from build123d import *

# Parameters (mm, degrees)
F1_R      = 300
F2_DEPTH  = 550
F3_R      = 200
F4_DEPTH  = 150
F5_R      = 100
F6_DEPTH  = 400.001
F8_DEPTH  = 250
F10_DEPTH = 250
F12_DEPTH = 250.001
F13_R     = 60
F14_DEPTH = 250.001


with BuildPart() as f2:
    # F1 (on Top) → F2 (new body)
    with BuildSketch(Plane.XY):
        Circle(F1_R)
    extrude(amount=F2_DEPTH)

    # F3 (on face) → F4 (cut)
    with BuildSketch(Plane.XY.offset(550)):
        Circle(F3_R)
    extrude(amount=-F4_DEPTH, mode=Mode.SUBTRACT)

    # F5 (on face) → F6 (cut, through all)
    with BuildSketch(Plane.XY.offset(400)):
        Circle(F5_R)
    extrude(amount=-F6_DEPTH, mode=Mode.SUBTRACT)

    # F7 (on face) → F8 (join)
    with BuildSketch(Plane(origin=(0, 0, 0), x_dir=(1, 0, 0), z_dir=(0, 0, -1))):
        with BuildLine():
            Line((-240, -180), (-240, 180))
            Line((-240, 180), (-540, 180))
            ThreePointArc((-540, 180), (-610.710678, 150.710678), (-640, 80))
            Line((-640, 80), (-640, -80))
            ThreePointArc((-640, -80), (-610.710678, -150.710678), (-540, -180))
            Line((-540, -180), (-240, -180))
        make_face()
    extrude(amount=-F8_DEPTH)

    # F9 (on face) → F10 (join)
    with BuildSketch(Plane(origin=(0, 0, 0), x_dir=(1, 0, 0), z_dir=(0, 0, -1))):
        with BuildLine():
            Line((540, 180), (240, 180))
            Line((240, 180), (240, -180))
            Line((240, -180), (540, -180))
            ThreePointArc((540, -180), (610.710678, -150.710678), (640, -80))
            Line((640, -80), (640, 80))
            ThreePointArc((640, 80), (610.710678, 150.710678), (540, 180))
        make_face()
    extrude(amount=-F10_DEPTH)

    # F11 (on face) → F12 (cut, through all)
    with BuildSketch(Plane.XY.offset(250)):
        with BuildLine():
            Line((430, 0), (550, 0))
            ThreePointArc((550, 0), (490, 60), (430, 0))
        make_face()
        with BuildLine():
            ThreePointArc((430, 0), (490, -60), (550, 0))
            Line((550, 0), (430, 0))
        make_face()
    extrude(amount=-F12_DEPTH, mode=Mode.SUBTRACT)

    # F13 (on face) → F14 (cut, through all)
    with BuildSketch(Plane.XY.offset(250)):
        with Locations((-490, 0)):
            Circle(F13_R)
    extrude(amount=-F14_DEPTH, mode=Mode.SUBTRACT)


solid = f2.part
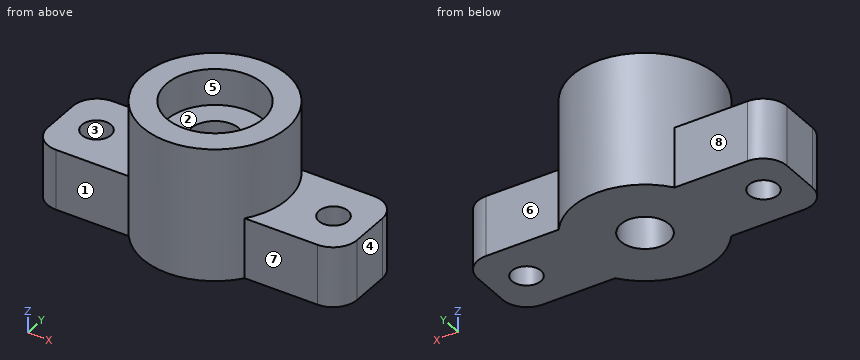
Here's how the part is built. I have some questions about the finished solid (model axes, mm). Face numbers are marked on the shaded views. A direction names the side the tool comes from. Round coordinates to 2 decimals unless told otherwise and drop trailing zeros. Order: outer loops, then holes, each group sorted by start corner. A loop starts at its lowest first (then second) coordinate and runs counter-clockwise, first axis right, second up. Notation, with made-up numbers: M 61,-6 L 79,-6 A19 ccw 79,13 Z; hole C -22.75,14 d1. An arc over 180 degrees is marked long. Return JSON: item names as keys, results as strings. Group by question number.
1. If we mould it in two halves opening along X, with no side actions, what happens to the marked faces 1, 2, 3 and 4? For each: pulls with the +X half, pulls with the -X half, needs draft (parallel to the pull), parting line crosses it, or undercut.
2. If we section it at B-B on x = 0: List the corners of the cut face in (y, z) for me, then the cut area to 3 significant figures.
3. On a 3-axis mill with a long thin cutter (end or side, diameter ignored), from which of +Z, -Z, +X, -X, +Y, -Y can I reach the whole of each face in a straight line? I mean the marked faces 5, 6, 7 and 8. Say none if no direction works.
4. If we section it at A-A on y = 0: List the corners of the cut face in (x, z) for me, then the cut area to 3 significant figures.
5. If we section it at C-C on z = 209: List the corners of the cut face in (x, y) for me, then the cut area to 3 significant figures.
6. I'm going to push flat-ended pins straight in: pin 1 Ø3 at (x, z) = (-395.5, 113.5) entering from +Y; pin 2 Ø12 at (x, z) = (-71.5, 76) entering from +Y; pin 3 Ø1 at (x, y) = (-386.5, -71.5) entering from +Z. Where does each tip first touch, or does it pass through?
7. Please list where these lines run through material, in increasing order: probe 1 along X at (y, z) = (5, 113); probe 2 along Y at (x, z) = (0, 433); probe 3 along X at (y, z) = (-17, 99).
8. If we section it at D-D on x = 490: List the corners of the cut face in (y, z) for me.
Reply:
{
 "1": {"face 1": "needs draft", "face 2": "undercut", "face 3": "undercut", "face 4": "pulls with the +X half"},
 "2": {"outline": "M -300,0 L -100,0 L -100,400 L -200,400 L -200,550 L -300,550 Z; M 100,0 L 300,0 L 300,550 L 200,550 L 200,400 L 100,400 Z", "area": "190,000 mm^2"},
 "3": {"face 5": "+Z", "face 6": "+Z, -Z, +X, +Y", "face 7": "+Z, -Z, +X, -Y", "face 8": "+Z, -Z, -X, +Y"},
 "4": {"outline": "M -640,0 L -550,0 L -550,250 L -640,250 Z; M -430,0 L -100,0 L -100,400 L -200,400 L -200,550 L -300,550 L -300,250 L -430,250 Z; M 100,0 L 430,0 L 430,250 L 300,250 L 300,550 L 200,550 L 200,400 L 100,400 Z; M 550,0 L 640,0 L 640,250 L 550,250 Z", "area": "300,000 mm^2"},
 "5": {"outline": "M -640,-80 A100 ccw -540,-180 L -240,-180 A300 ccw 240,-180 L 540,-180 A100 ccw 640,-80 L 640,80 A100 ccw 540,180 L 240,180 A300 ccw -240,180 L -540,180 A100 ccw -640,80 Z; hole C -490,0 d120; hole C 0,0 d200; hole C 490,0 d120", "area": "479,000 mm^2"},
 "6": {"pin 1": "y = 180", "pin 2": "y = 292.76", "pin 3": "z = 250"},
 "7": {"probe 1": "-640 to -549.79, -430.21 to -99.87, 99.87 to 430.21, 549.79 to 640", "probe 2": "-300 to -200, 200 to 300", "probe 3": "-640 to -547.54, -432.46 to -98.54, 98.54 to 432.46, 547.54 to 640"},
 "8": {"outline": "M -180,0 L -60,0 L -60,250 L -180,250 Z; M 60,0 L 180,0 L 180,250 L 60,250 Z"}
}
